The drawing under review shows one solid part. Ordinate dimensions are in mm from its lowest x, y, z. A direction names the side the tool comes from. Coordinates: 2 decimals unless noted, no trailing zeros. Order: outer loops, then holes, each group sorted by start corner. A loop starts at its lowest first (then second) coordinate and runs counter-clockwise, first axis right, second up. Notation, with made-up numbers: M 46.5,-32.75 L 99.5,-32.75 A12 ccw 99.5,-19.75 Z; hole C -21.5,33.25 d2. An arc over 180 degrees is marked long. Answer as a JSON object with one key per item and string values.
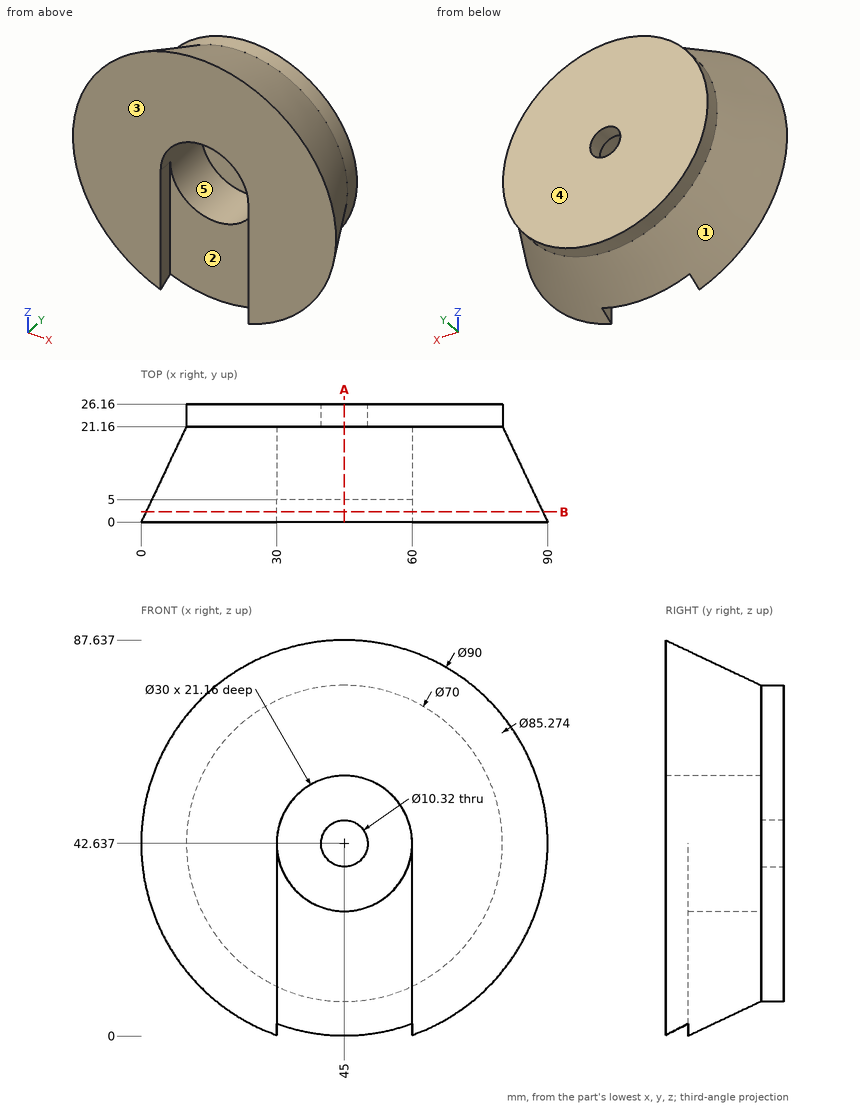
1) Mouldability with a two-part tool opening along X and no side actions: class the marked faces 1, 2 and 3 as released by +X, released by -X, zero draft, split by the parting line, or undercut.
Taken from the geometry:
{"face 1": "split by the parting line", "face 2": "undercut", "face 3": "zero draft"}
2) Tool access review of the marked faces 4 and 5: name each direction out of +Z, -Z, +X, -X, +Y, -Y from which nothing blocks a thin tool from reaching the whole face with its end or side.
Taken from the geometry:
{"face 4": "+Z, -Z, +X, -X, +Y", "face 5": "-Y"}
3) Insertion check: pin 1 Ø4 at (x, z) = (16, 72) entering from +Y (1 decimal); pin 2 Ø4 at (y, z) = (13.5, 61) entering from +X; pin 3 Ø4 at (y, z) = (3, 28.5) entering from -X; pin 4 Ø24 at (x, z) = (51.5, 23) entering from -Y. Each pin has a flat end and moves straight along its axis. Give the tip position at first contact, or say it passes through.
Taken from the geometry:
{"pin 1": "stops at y = 12.1", "pin 2": "stops at x = 80.45", "pin 3": "stops at x = 2.59", "pin 4": "stops at y = 0"}
4) To check wall thickness, follow L1, parallel to X at y = 14.25, z = 32.5; L2, parallel to Z at x = 42.5, y = 25.25; L3, parallel to Y at x = 57, z = 17. State the ranges of each line that lie inside material, in increasing order.
Taken from the geometry:
{"L1": "x = 8.1 to 33.94, 56.06 to 81.9", "L2": "z = 7.73 to 38.12, 47.15 to 77.55", "L3": "y = 5 to 26.16"}
5) Add section A-A (x = 45). State the section outline as (y, z) points, and give its area (3 significant figures).
Taken from the geometry:
{"outline": "M 0,57.64 L 21.16,57.64 L 21.16,47.8 L 26.16,47.8 L 26.16,77.64 L 21.16,77.64 L 0,87.64 Z; M 5,0 L 21.16,7.64 L 26.16,7.64 L 26.16,37.48 L 21.16,37.48 L 21.16,27.64 L 5,27.64 Z", "area": "1,210 mm2"}
6) Add section B-B (y = 2.25). State the section outline as (x, z) points.
Taken from the geometry:
{"outline": "M 30,1.34 L 30,42.64 A15 cw 60,42.64 L 60,1.34 A43.94 ccw long Z"}
